Input: part model. Units: mm. Frame: model coordinates. Face numbers are marked on the shaded views. A direction names the side the tool comes from. Coordinates: 2 decimals unless noted, no trailing zeros. Order: outer loops, then holes, each group sorted by start corner. A loop starts at its lowest first (then second) coordinate and runs counter-clockwise, first axis right, second up. Notation, with made-up numbers: M -5.75,-2.5 L 16.25,-2.5 A13 cw 16.25,8.5 Z; hole C -13.75,1.5 d1. An arc over 180 degrees is marked long. Answer in a Markdown table with one row per item.
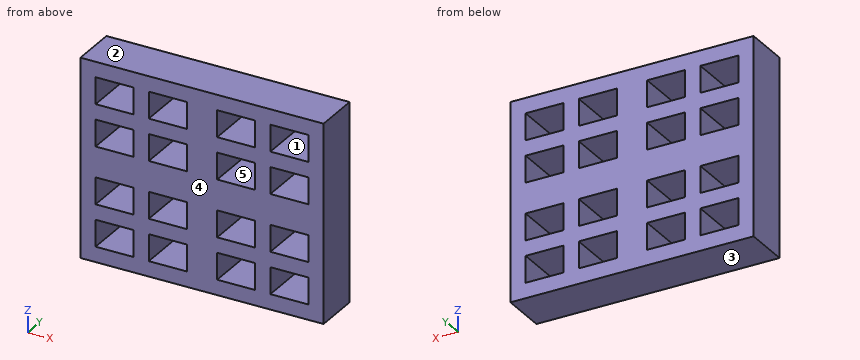
from build123d import *

# Parameters (mm, degrees)
SKETCH1_W           = 16
SKETCH1_H           = 13
SKETCH1_W_2         = 2.5
SKETCH1_H_2         = 1.75
BOSS_EXTRUDE1_DEPTH = 3


with BuildPart() as part:
    # Sketch1 → Boss-Extrude1 (new body)
    with BuildSketch(Plane(origin=(0, 0, 0), x_dir=(1, 0, 0), z_dir=(0, 1, 0))):
        with Locations((-4.357364788, -0.36440678)):
            Rectangle(SKETCH1_W, SKETCH1_H)
        with Locations((-10.107364788, 1.51059322)):
            Rectangle(SKETCH1_W_2, SKETCH1_H_2, mode=Mode.SUBTRACT)
        with Locations((-10.107364788, 4.26059322)):
            Rectangle(SKETCH1_W_2, SKETCH1_H_2, mode=Mode.SUBTRACT)
        with Locations((-6.607364788, 1.51059322)):
            Rectangle(SKETCH1_W_2, SKETCH1_H_2, mode=Mode.SUBTRACT)
        with Locations((-6.607364788, 4.26059322)):
            Rectangle(SKETCH1_W_2, SKETCH1_H_2, mode=Mode.SUBTRACT)
        with Locations((-6.607364788, -2.23940678)):
            Rectangle(SKETCH1_W_2, SKETCH1_H_2, mode=Mode.SUBTRACT)
        with Locations((-10.107364788, -2.23940678)):
            Rectangle(SKETCH1_W_2, SKETCH1_H_2, mode=Mode.SUBTRACT)
        with Locations((-6.607364788, -4.98940678)):
            Rectangle(SKETCH1_W_2, SKETCH1_H_2, mode=Mode.SUBTRACT)
        with Locations((-10.107364788, -4.98940678)):
            Rectangle(SKETCH1_W_2, SKETCH1_H_2, mode=Mode.SUBTRACT)
        with Locations((-2.107364788, -4.98940678)):
            Rectangle(SKETCH1_W_2, SKETCH1_H_2, mode=Mode.SUBTRACT)
        with Locations((1.392635212, -4.98940678)):
            Rectangle(SKETCH1_W_2, SKETCH1_H_2, mode=Mode.SUBTRACT)
        with Locations((-2.107364788, -2.23940678)):
            Rectangle(SKETCH1_W_2, SKETCH1_H_2, mode=Mode.SUBTRACT)
        with Locations((1.392635212, -2.23940678)):
            Rectangle(SKETCH1_W_2, SKETCH1_H_2, mode=Mode.SUBTRACT)
        with Locations((-2.107364788, 1.51059322)):
            Rectangle(SKETCH1_W_2, SKETCH1_H_2, mode=Mode.SUBTRACT)
        with Locations((1.392635212, 1.51059322)):
            Rectangle(SKETCH1_W_2, SKETCH1_H_2, mode=Mode.SUBTRACT)
        with Locations((-2.107364788, 4.26059322)):
            Rectangle(SKETCH1_W_2, SKETCH1_H_2, mode=Mode.SUBTRACT)
        with Locations((1.392635212, 4.26059322)):
            Rectangle(SKETCH1_W_2, SKETCH1_H_2, mode=Mode.SUBTRACT)
    extrude(amount=BOSS_EXTRUDE1_DEPTH)


solid = part.part
1) Cut plane B-B, the plane x = 2.25. Output: boundary loops of the cut face in (y, z), and give its area (3 significant figures).
Resolved:
| item | result |
|---|---|
| outline | M 0,-6.14 L 3,-6.14 L 3,-5.14 L 0,-5.14 Z; M 0,-3.39 L 3,-3.39 L 3,-2.39 L 0,-2.39 Z; M 0,-0.64 L 3,-0.64 L 3,1.36 L 0,1.36 Z; M 0,3.11 L 3,3.11 L 3,4.11 L 0,4.11 Z; M 0,5.86 L 3,5.86 L 3,6.86 L 0,6.86 Z |
| area | 18.0 mm2 |
2) Mould query, pull axis Z, two halves, no side actions, for the marked faces 1, 2 and 3. Classes: +Z half, -Z half, draft (parallel to the pull), parting line (faces both ways), or undercut.
Resolved:
| item | result |
|---|---|
| face 1 | undercut |
| face 2 | +Z half |
| face 3 | -Z half |
3) Cut plane C-C, the plane y = 0.45. State how many separate pieces and enclosed holes the cut face has, and give its area (3 significant figures).
Resolved:
| item | result |
|---|---|
| separate pieces | 1 |
| enclosed holes | 16 |
| area | 138 mm2 |
4) Cut plane A-A, the plane z = 4.75. Output: boundary loops of the cut face in (x, y), and give its area (3 significant figures).
Resolved:
| item | result |
|---|---|
| outline | M -12.36,0 L -11.36,0 L -11.36,3 L -12.36,3 Z; M -8.86,0 L -7.86,0 L -7.86,3 L -8.86,3 Z; M -5.36,0 L -3.36,0 L -3.36,3 L -5.36,3 Z; M -0.86,0 L 0.14,0 L 0.14,3 L -0.86,3 Z; M 2.64,0 L 3.64,0 L 3.64,3 L 2.64,3 Z |
| area | 18.0 mm2 |
5) Reachability of the marked faces 4 and 5 from +Z, -Z, +X, -X, +Y, -Y: full face, straight path, thin tool, end or side. Return the list, or none.
Resolved:
| item | result |
|---|---|
| face 4 | +Z, -Z, +X, -X, -Y |
| face 5 | +Y, -Y |
6) Material intervals for probe 1 along Z at (x, y) = (1.5, 2.15); probe 2 along X at (y, z) = (2.1, -3.5), sorted ascending.
Resolved:
| item | result |
|---|---|
| probe 1 | z = -6.14 to -5.14, -3.39 to -2.39, -0.64 to 1.36, 3.11 to 4.11, 5.86 to 6.86 |
| probe 2 | x = -12.36 to -11.36, -8.86 to -7.86, -5.36 to -3.36, -0.86 to 0.14, 2.64 to 3.64 |
